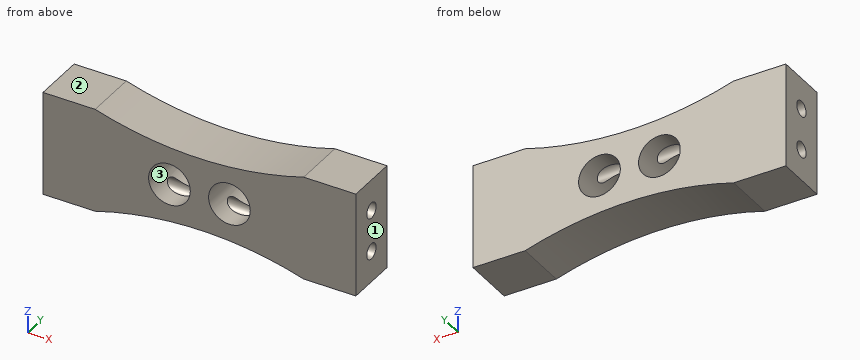
from build123d import *

# Parameters (mm, degrees)
F0_R     = 4
F1_DEPTH = 10
F2_R     = 1.5
F3_DEPTH = 60


with BuildPart() as f1:
    # F0 (on Front) → F1 (new body)
    with BuildSketch(Plane.XZ):
        with BuildLine():
            Line((-30, 10), (-30, -10))
            Line((-30, -10), (-20, -10))
            ThreePointArc((-20, -10), (0, -7), (20, -10))
            Line((20, -10), (30, -10))
            Line((30, -10), (30, 10))
            Line((30, 10), (20, 10))
            ThreePointArc((20, 10), (0, 7), (-20, 10))
            Line((-20, 10), (-30, 10))
        make_face()
        with Locations((-5.75, 0)):
            Circle(F0_R, mode=Mode.SUBTRACT)
        with Locations((5.75, 0)):
            Circle(F0_R, mode=Mode.SUBTRACT)
    extrude(amount=F1_DEPTH)

    # F2 (on face) → F3 (cut)
    with BuildSketch(Plane.YZ.offset(30)):
        with Locations((-5, 4)):
            Circle(F2_R)
        with Locations((-5, -4)):
            Circle(F2_R)
    extrude(amount=-F3_DEPTH, mode=Mode.SUBTRACT)


solid = f1.part
Source: CAD feature listing. Evaluate the final solid. Frame: model axes, mm. Face numbers are marked on the shaded views. Round coordinates to 2 decimals unless told otherwise and drop trailing zeros. Order: outer loops, then holes, each group sorted by start corner. A loop starts at its lowest first (then second) coordinate and runs counter-clockwise, first axis right, second up. Notation, with made-up numbers: (-29, 49) - (28, 49) arc R15 ccw to (28, 69) - close; hole circle Ø11 at (69, -34.75). An arc over 180 degrees is marked (long way). Use a Markdown table: item, result. Add a question column.
1. First-contact query: pin 1 (6 mm diameter, centred on x = 14.5, z = 5, fed in from +Y); pin 2 (5 mm diameter, centred on x = -14, y = -5.5, fed in from -Z). Flat tips, straight axial feed; report the tip coordinate or a pass-through.
2. Section query A-A (y = -1). Return the cut outline in (x, z).
3. Section query C-C (x = 21). Return the cut outline in (y, z).
4. Section query B-B (z = -0.75). Return the cut outline in (x, y), then the cut area to 3 significant figures.
5. Mould query, pull axis Z, two halves, no side actions, for the marked faces 1, 2 and 3. Classes: +Z half, -Z half, draft (parallel to the pull), parting line (faces both ways), or undercut.
6. Section query D-D (y = -5). Return the cut outline in (x, z), then the cut area to 3 significant figures.
7. Line query: probe 1 along Z at (x, y) = (0.5, -5); probe 2 along X at (y, z) = (-3.5, 0.25); probe 3 along Z at (x, y) = (-11.5, -6). Output: solid intervals per line, ascending.
Derived:
| question | item | result |
|---|---|---|
| 1 | pin 1 | y = 0 |
| 1 | pin 2 | z = -9.03 |
| 2 | outline | (-30, -10) - (-20, -10) arc R68.17 cw to (20, -10) - (30, -10) - (30, 10) - (20, 10) arc R68.17 cw to (-20, 10) - (-30, 10) - close; hole circle Ø8 at (-5.75, 0); hole circle Ø8 at (5.75, 0) |
| 3 | outline | (-10, -10) - (0, -10) - (0, 10) - (-10, 10) - close; hole circle Ø3 at (-5, -4); hole circle Ø3 at (-5, 4) |
| 4 | outline | (-30, -10) - (-9.68, -10) - (-9.68, 0) - (-30, 0) - close; (-1.82, -10) - (1.82, -10) - (1.82, 0) - (-1.82, 0) - close; (9.68, -10) - (30, -10) - (30, 0) - (9.68, 0) - close |
| 4 | area | 443 mm2 |
| 5 | face 1 | draft |
| 5 | face 2 | +Z half |
| 5 | face 3 | undercut |
| 6 | outline | (-30, -10) - (-20, -10) arc R68.17 cw to (20, -10) - (30, -10) - (30, -5.5) - (-30, -5.5) - close; (-30, -2.5) - (-8.87, -2.5) arc R4 cw to (-8.87, 2.5) - (-30, 2.5) - close; (-30, 5.5) - (30, 5.5) - (30, 10) - (20, 10) arc R68.17 cw to (-20, 10) - (-30, 10) - close; (-2.63, -2.5) - (2.63, -2.5) arc R4 cw to (2.63, 2.5) - (-2.63, 2.5) arc R4 cw to start; (8.87, -2.5) - (30, -2.5) - (30, 2.5) - (8.87, 2.5) arc R4 cw to start |
| 6 | area | 605 mm2 |
| 7 | probe 1 | -7 to -5.5, -2.5 to 2.5, 5.5 to 7 |
| 7 | probe 2 | -30 to -9.74, -1.76 to 1.76, 9.74 to 30 |
| 7 | probe 3 | -7.98 to -5.12, -2.88 to 2.88, 5.12 to 7.98 |
